from build123d import *

# Parameters (mm, degrees)
PAD_DEPTH    = 4
SKETCH001_R  = 1.8
POCKET_DEPTH = 5


with BuildPart() as part:
    # Sketch → Pad (new body)
    with BuildSketch(Plane.XY):
        Polygon((-66, 0), (-66, 36), (66, 36), (66, 0), (26, 0), (26, -60), (-26, -60), (-26, 0), align=None)
    extrude(amount=PAD_DEPTH)

    # Sketch001 (on Face10 of Pad) → Pocket (cut)
    with BuildSketch(Plane.XY.offset(4)):
        with Locations((-60, 28)):
            Circle(SKETCH001_R)
        with Locations((-40, 28)):
            Circle(SKETCH001_R)
        with Locations((-60, 8)):
            Circle(SKETCH001_R)
        with Locations((-40, 8)):
            Circle(SKETCH001_R)
        with Locations((40, 28)):
            Circle(SKETCH001_R)
        with Locations((40, 8)):
            Circle(SKETCH001_R)
        with Locations((60, 28)):
            Circle(SKETCH001_R)
        with Locations((60, 8)):
            Circle(SKETCH001_R)
        with Locations((-20, -52)):
            Circle(SKETCH001_R)
        with Locations((0, -52)):
            Circle(SKETCH001_R)
        with Locations((20, -52)):
            Circle(SKETCH001_R)
        with Locations((-20, -32)):
            Circle(SKETCH001_R)
        with Locations((0, -32)):
            Circle(SKETCH001_R)
        with Locations((20, -32)):
            Circle(SKETCH001_R)
        with Locations((-20, -12)):
            Circle(SKETCH001_R)
        with Locations((0, -12)):
            Circle(SKETCH001_R)
        with Locations((20, -12)):
            Circle(SKETCH001_R)
        with Locations((20, 8)):
            Circle(SKETCH001_R)
        with Locations((0, 8)):
            Circle(SKETCH001_R)
        with Locations((-20, 8)):
            Circle(SKETCH001_R)
        with Locations((-20, 28)):
            Circle(SKETCH001_R)
        with Locations((0, 28)):
            Circle(SKETCH001_R)
        with Locations((20, 28)):
            Circle(SKETCH001_R)
    extrude(amount=-POCKET_DEPTH, mode=Mode.SUBTRACT)


solid = part.part
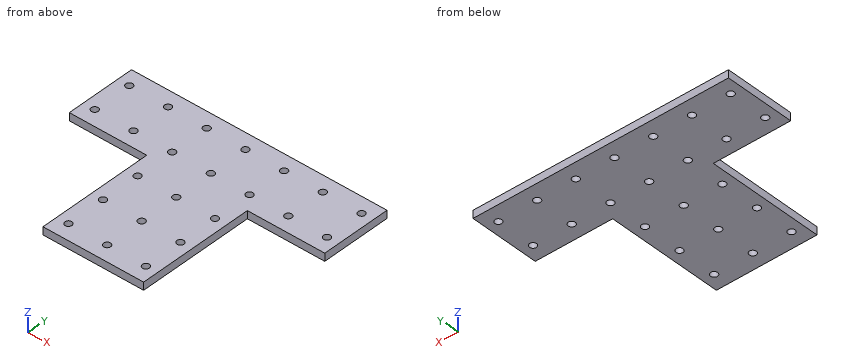
Work out the finished part from the listing and answer in its coordinate system (mm). Give positions to 0.01 mm unless a question says otherwise; leave off trailing zeros. Loops run counter-clockwise (first coordinate to the right, second up) from the corner with the lowest first, then second, coordinate; pieces in that order, holes last. Notation, with made-up numbers: (1, -10.5) - (39, -10.5) arc R26 cw to (39, 27.5) - close; hole circle Ø3 at (16.5, 30.5). An arc over 180 degrees is marked (long way). Answer in a Markdown table with one row per item.
(1) Flat-ended cylindrical pins translate along their axes: pin 1 Ø6 at (x, y) = (-60, 8) entering from +Z; pin 2 Ø1.5 at (x, z) = (31.5, 3) entering from -Y; pin 3 Ø1.2 at (y, z) = (-34, 2) entering from +X. Find the tip coordinate at first contact, or state that the pin passes through.
Results list:
| item | result |
|---|---|
| pin 1 | stops at z = 4 |
| pin 2 | stops at y = 0 |
| pin 3 | stops at x = 26 |
(2) Section C-C (y = -32) is taken. Give the vertices of the cut face in (x, z).
Results list:
| item | result |
|---|---|
| outline | (-26, 0) - (-21.8, 0) - (-21.8, 4) - (-26, 4) - close; (-18.2, 0) - (-1.8, 0) - (-1.8, 4) - (-18.2, 4) - close; (1.8, 0) - (18.2, 0) - (18.2, 4) - (1.8, 4) - close; (21.8, 0) - (26, 0) - (26, 4) - (21.8, 4) - close |
(3) Section B-B (x = 40) is taken. Give the vertices of the cut face in (y, z), and give its area (3 significant figures).
Results list:
| item | result |
|---|---|
| outline | (0, 0) - (6.2, 0) - (6.2, 4) - (0, 4) - close; (9.8, 0) - (26.2, 0) - (26.2, 4) - (9.8, 4) - close; (29.8, 0) - (36, 0) - (36, 4) - (29.8, 4) - close |
| area | 115 mm² |
(4) Consider L1, parallel to Y at x = -20, z = 2.2; L2, parallel to X at y = -53.5, z = 0.8; L3, parallel to Y at x = -40, z = 2. Determine where each line is inside the solid, lowest interval first. Write a range as [from, to].
Results list:
| item | result |
|---|---|
| L1 | y = [-60, -53.8], [-50.2, -33.8], [-30.2, -13.8], [-10.2, 6.2], [9.8, 26.2], [29.8, 36] |
| L2 | x = [-26, -20.99], [-19.01, -0.99], [0.99, 19.01], [20.99, 26] |
| L3 | y = [0, 6.2], [9.8, 26.2], [29.8, 36] |
(5) Section A-A (y = 28) is taken. State how many separate pieces and enclosed holes the cut face has, and give its area (3 significant figures).
Results list:
| item | result |
|---|---|
| separate pieces | 8 |
| enclosed holes | 0 |
| area | 427 mm² |
